Geometry: final body of the model. Coordinates: model frame, mm. A direction names the side the tool comes from. Coordinates: 2 decimals unless noted, no trailing zeros. Order: outer loops, then holes, each group sorted by start corner. A loop starts at its lowest first (then second) coordinate and runs counter-clockwise, first axis right, second up. Notation, with made-up numbers: (-20.75, -3.5) -> (25.25, -3.5) arc R35 cw to (25.25, 32.5) -> close; hole circle Ø8 at (3.25, -9.5). An arc over 180 degrees is marked (long way). Answer in a Markdown table with one row per item. Add a question column.
1) Section query A-A on x = 0. Return the cut outline in (y, z), then the cut area to 3 significant figures.
2) Contact query for flat-ended pins moving along their axis: P1, Ø1.5, axis at y = 2.5, z = -1.5, coming from the -X side; P2, Ø1.5, axis at x = -7.5, z = 6, coming from the -Y side. Output: stop coordinate, or through.
3) Section query C-C on y = 1. Return the cut outline in (x, z).
4) Section query D-D on z = -8. Return the cut outline in (x, y).
5) Pull-direction query (Z, two-part tool) for faces 4 (the face through (11, -4, -5)), 5 (the face through (7.91, 0.056, -10.316)), 6 (the face through (3.955, -3.746, -5.158)), 7 (the face through (5, -3.5, 5)); classes: +Z half, -Z half, draft (parallel to the pull), parting line (faces both ways), or undercut.
6) Ray query, line 1 (X direction, y = -3.6, z = 0); line 2 (Z direction, x = 3.75, y = 1.25); line 3 (X direction, y = 2.5, z = -1). Return the intervals inside material, ascending. Write a range as from..to.
7) Section query B-B on z = 0. Return the cut outline in (x, y).
8) Set-up query: faces 1 (the face through (5, 3.5, 5)), 2 (the face through (-11.4, -3.7, -1.5)), 3 (the face through (5, 4, -2)). Return all of +Z, -Z, +X, -X, +Y, -Y with unobstructed straight access to the full face (end or side cutting, diameter ignored); none if empty.
```python
from build123d import *

# Parameters (mm, degrees)
ESBO_O1_W = 1.5
ESBO_O1_H = 8
ESBO_O4_W = 5
ESBO_O4_H = 7


with BuildPart() as part:
    # Esboço1 → Revolução1 (revolve)
    with BuildSketch(Plane.XY, mode=Mode.PRIVATE) as revolu_o1_sk:
        with Locations((5.75, 0)):
            Rectangle(ESBO_O1_W, ESBO_O1_H)
        with Locations((12.25, 0)):
            Rectangle(ESBO_O1_W, ESBO_O1_H)
    revolve(revolu_o1_sk.sketch.rotate(Axis((0, 7.601094967, 0), (0, -1, 0)), 90), axis=Axis((0, 7.601094967, 0), (0, -1, 0)))

    # Esboço4 → Revolução2 (revolve)
    with BuildSketch(Plane.XY, mode=Mode.PRIVATE) as revolu_o2_sk:
        with Locations((-9, 0)):
            Rectangle(ESBO_O4_W, ESBO_O4_H)
    revolve(revolu_o2_sk.sketch.rotate(Axis((0, 5.982287702, 0), (0, -1, 0)), 270), axis=Axis((0, 5.982287702, 0), (0, -1, 0)))


solid = part.part
```
Result:
| question | item | result |
|---|---|---|
| 1 | outline | (-4, -13) -> (4, -13) -> (4, -11.5) -> (3.5, -11.5) -> (3.5, -6.5) -> (4, -6.5) -> (4, -5) -> (-4, -5) -> (-4, -6.5) -> (-3.5, -6.5) -> (-3.5, -11.5) -> (-4, -11.5) -> close; (-4, 5) -> (4, 5) -> (4, 6.5) -> (3.5, 6.5) -> (3.5, 11.5) -> (4, 11.5) -> (4, 13) -> (-4, 13) -> (-4, 11.5) -> (-3.5, 11.5) -> (-3.5, 6.5) -> (-4, 6.5) -> close |
| 1 | area | 118 mm2 |
| 2 | P1 | x = -12.98 |
| 2 | P2 | y = -3.5 |
| 3 | outline | circle Ø26 at (0, 0); hole circle Ø10 at (0, 0) |
| 4 | outline | (-10.25, -4) -> (-8.26, -4) -> (-8.26, -3.5) -> (8.26, -3.5) -> (8.26, -4) -> (10.25, -4) -> (10.25, 4) -> (8.26, 4) -> (8.26, 3.5) -> (-8.26, 3.5) -> (-8.26, 4) -> (-10.25, 4) -> close |
| 5 | face 4 | draft |
| 5 | face 5 | parting line |
| 5 | face 6 | undercut |
| 5 | face 7 | undercut |
| 6 | line 1 | -13..-11.5, -6.5..-5, 5..6.5, 11.5..13 |
| 6 | line 2 | -12.45..-3.31, 3.31..12.45 |
| 6 | line 3 | -12.96..-4.9, 4.9..12.96 |
| 7 | outline | (-13, -4) -> (-11.5, -4) -> (-11.5, -3.5) -> (-6.5, -3.5) -> (-6.5, -4) -> (-5, -4) -> (-5, 4) -> (-6.5, 4) -> (-6.5, 3.5) -> (-11.5, 3.5) -> (-11.5, 4) -> (-13, 4) -> close; (5, -4) -> (6.5, -4) -> (6.5, -3.5) -> (11.5, -3.5) -> (11.5, -4) -> (13, -4) -> (13, 4) -> (11.5, 4) -> (11.5, 3.5) -> (6.5, 3.5) -> (6.5, 4) -> (5, 4) -> close |
| 8 | face 1 | +Y |
| 8 | face 2 | -Y |
| 8 | face 3 | +Z, -Z, +X, -X, +Y |
